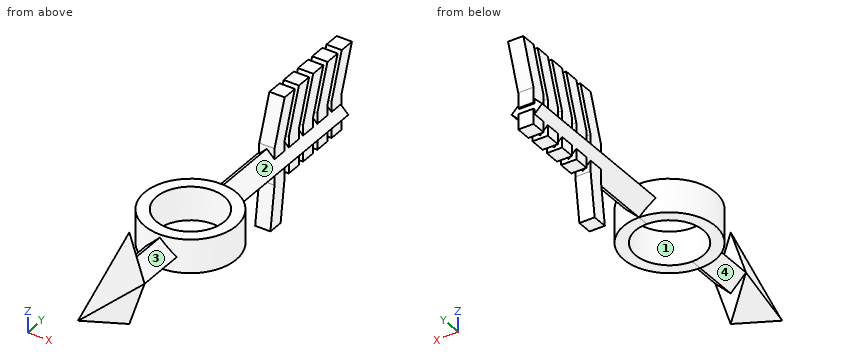
from build123d import *

# Parameters (mm, degrees)
F2_R       = 0.1
F5_DEPTH   = 100
F7_R       = 15
F7_R_2     = 11
F8_DEPTH   = 11
F9_R       = 11.1
F10_DEPTH  = 21.001
F11_W      = 5
F11_H      = 5
F14_DEPTH  = 5
F14_FACE_W = 5
F14_FACE_H = 5
F13_W      = 5
F13_H      = 5
F21_W      = 5
F21_H      = 5
F22_DEPTH  = 5
F22_FACE_W = 5
F22_FACE_H = 5
F24_W      = 5
F24_H      = 5


with BuildPart() as f3:
    # F0 (on Front) → F3 section 0
    with BuildSketch(Plane.XZ):
        Polygon((5, 0), (0, 15), (-5, 0), (0, -15), align=None)
    # F2 (on offset) → F3 section 1
    with BuildSketch(Plane.XZ.offset(25)):
        Circle(F2_R)
    loft()

    # F4 (on Front) → F5 (join)
    with BuildSketch(Plane.XZ):
        Polygon((2e-06, 5.000002), (-5, 0), (2e-06, -5.000002), (5.000005, 0), align=None)
    extrude(amount=-F5_DEPTH)

    # F7 (on offset) → F8 (join)
    with BuildSketch(Plane.XY.offset(6)):
        with Locations((0, 30)):
            Circle(F7_R)
        with Locations((0, 30)):
            Circle(F7_R_2, mode=Mode.SUBTRACT)
    extrude(amount=-F8_DEPTH)

    # F9 (on offset) → F10 (cut, through all)
    with BuildSketch(Plane.XY.offset(6)):
        with Locations((0, 30)):
            Circle(F9_R)
    extrude(amount=-F10_DEPTH, mode=Mode.SUBTRACT)

    # F11 (on offset) → F14 (join)
    with BuildSketch(Plane.XY.offset(6)):
        with Locations((0, 70)):
            Rectangle(F11_W, F11_H)
        with Locations((0, 77)):
            Rectangle(F11_W, F11_H)
        with Locations((0, 84)):
            Rectangle(F11_W, F11_H)
        with Locations((0, 91)):
            Rectangle(F11_W, F11_H)
        with Locations((0, 98)):
            Rectangle(F11_W, F11_H)
    extrude(amount=-F14_DEPTH)

    # F14_face (on face) → F15 section 0
    with BuildSketch(Plane(origin=(0, 70, 6), x_dir=(1, 0, 0), z_dir=(0, 0, 1))):
        Rectangle(F14_FACE_W, F14_FACE_H)
    # F13 (on offset) → F15 section 1
    with BuildSketch(Plane.XY.offset(20)):
        with Locations((0, 75)):
            Rectangle(F13_W, F13_H)
    loft()

    # F14_face (on face) → F16 section 0
    with BuildSketch(Plane(origin=(0, 70, 6), x_dir=(1, 0, 0), z_dir=(0, 0, 1))):
        with Locations((0, 7)):
            Rectangle(F14_FACE_W, F14_FACE_H)
    # F13 (on offset) → F16 section 1
    with BuildSketch(Plane.XY.offset(20)):
        with Locations((0, 82)):
            Rectangle(F13_W, F13_H)
    loft()

    # F14_face (on face) → F17 section 0
    with BuildSketch(Plane(origin=(0, 70, 6), x_dir=(1, 0, 0), z_dir=(0, 0, 1))):
        with Locations((0, 14)):
            Rectangle(F14_FACE_W, F14_FACE_H)
    # F13 (on offset) → F17 section 1
    with BuildSketch(Plane.XY.offset(20)):
        with Locations((0, 89)):
            Rectangle(F13_W, F13_H)
    loft()

    # F14_face (on face) → F18 section 0
    with BuildSketch(Plane(origin=(0, 70, 6), x_dir=(1, 0, 0), z_dir=(0, 0, 1))):
        with Locations((0, 21)):
            Rectangle(F14_FACE_W, F14_FACE_H)
    # F13 (on offset) → F18 section 1
    with BuildSketch(Plane.XY.offset(20)):
        with Locations((0, 96)):
            Rectangle(F13_W, F13_H)
    loft()

    # F14_face (on face) → F19 section 0
    with BuildSketch(Plane(origin=(0, 70, 6), x_dir=(1, 0, 0), z_dir=(0, 0, 1))):
        with Locations((0, 28)):
            Rectangle(F14_FACE_W, F14_FACE_H)
    # F13 (on offset) → F19 section 1
    with BuildSketch(Plane.XY.offset(20)):
        with Locations((0, 103)):
            Rectangle(F13_W, F13_H)
    loft()

    # F21 (on offset) → F22 (join)
    with BuildSketch(Plane.XY.offset(-6)):
        with Locations((0, 70)):
            Rectangle(F21_W, F21_H)
        with Locations((0, 77)):
            Rectangle(F21_W, F21_H)
        with Locations((0, 84)):
            Rectangle(F21_W, F21_H)
        with Locations((0, 91)):
            Rectangle(F21_W, F21_H)
        with Locations((0, 98)):
            Rectangle(F21_W, F21_H)
    extrude(amount=F22_DEPTH)

    # F22_face (on face) → F25 section 0
    with BuildSketch(Plane(origin=(0, 70, -6), x_dir=(1, 0, 0), z_dir=(0, 0, -1))):
        Rectangle(F22_FACE_W, F22_FACE_H)
    # F24 (on offset) → F25 section 1
    with BuildSketch(Plane.XY.offset(-20)):
        with Locations((0, 68)):
            Rectangle(F24_W, F24_H)
    loft()


solid = f3.part
Geometry check sheet. Reference: the model listing, model coordinates, mm. Face numbers are marked on the shaded views. A direction names the side the tool comes from. Give positions to 0.01 mm unless a question says otherwise; leave off trailing zeros. Order: outer loops, then holes, each group sorted by start corner. A loop starts at its lowest first (then second) coordinate and runs counter-clockwise, first axis right, second up. Notation, with made-up numbers: (8, 30) - (17, 30) arc R37 ccw to (17, 69) - close; hole circle Ø6 at (61.25, 23.25). An arc over 180 degrees is marked (long way). Use one line per item in the form item = value.
1) Sectioned sample at A-A (y = 30). Record the boundary of the cut face in (x, z).
Working result:
outline = (-15, -5) - (-11.1, -5) - (-11.1, 6) - (-15, 6) - close; (11.1, -5) - (15, -5) - (15, 6) - (11.1, 6) - close
2) Sectioned sample at C-C (y = 76). Record the boundary of the cut face in (x, z).
Working result:
outline = (-5, 0) - (-2.5, -2.5) - (-2.5, -6) - (2.5, -6) - (2.5, -2.5) - (5, 0) - (2.5, 2.5) - (2.5, 10.2) - (-2.5, 10.2) - (-2.5, 2.5) - close; (-2.5, 15.8) - (2.5, 15.8) - (2.5, 20) - (-2.5, 20) - close
3) Depth check by flat-ended pin: pin 1 Ø4 at (x, z) = (-0.5, 4) entering from -Y; pin 2 Ø8 at (y, z) = (70, 9.5) entering from +X; pin 3 Ø4 at (x, z) = (-1, -5) entering from -Y. Enter the tip coordinate at first touch or a pass-through.
Working result:
pin_1 = -21.71
pin_2 = 2.5
pin_3 = -19.68
4) Material ranges on probe 1 along X at (y, z) = (30, -1); probe 2 along X at (y, z) = (99, 6.5); probe 3 along Z at (x, y) = (-4.5, 44), recorded low to high. Write a range as from..to.
Working result:
probe_1 = -15..-11.1, 11.1..15
probe_2 = -2.5..2.5
probe_3 = -5..6
5) Sectioned sample at D-D (z = 11). Count the separate pieces of the cut face and the enclosed holes in it, and give its area (3 significant figures).
Working result:
separate_pieces = 6
enclosed_holes = 0
area = 134 mm^2
6) Draft check along Y on the marked faces 1 and 2. Enter one of: released by +Y, released by -Y, zero draft, split by the parting line, or undercut.
Working result:
face_1 = undercut
face_2 = undercut
7) Access from +Z, -Z, +X, -X, +Y, -Y to the whole of each face (thin tool, end or side, straight path). Record for the marked faces 3 and 4.
Working result:
face_3 = +Z, +X
face_4 = -Z, -X
8) Sectioned sample at B-B (x = -7.25). Record the boundary of the cut face in (y, z).
Working result:
outline = (16.87, -5) - (21.59, -5) - (21.59, 6) - (16.87, 6) - close; (38.41, -5) - (43.13, -5) - (43.13, 6) - (38.41, 6) - close
